from build123d import *

# Parameters (mm, degrees)
SKETCH1_R           = 61.976
SKETCH1_R_2         = 12.827
BOSS_EXTRUDE1_DEPTH = 45.974
SKETCH2_R           = 60.325
CUT_EXTRUDE1_DEPTH  = 20.32


with BuildPart() as part:
    # Sketch1 → Boss-Extrude1 (new body)
    with BuildSketch(Plane.XY):
        Circle(SKETCH1_R)
        Circle(SKETCH1_R_2, mode=Mode.SUBTRACT)
    extrude(amount=BOSS_EXTRUDE1_DEPTH)

    # Sketch2 → Cut-Extrude1 (cut)
    with BuildSketch(Plane.XY):
        Circle(SKETCH2_R)
    cut_extrude1 = extrude(amount=CUT_EXTRUDE1_DEPTH, mode=Mode.SUBTRACT)

    # Mirror1: Cut-Extrude1 across plane
    add(cut_extrude1.mirror(Plane.XY.offset(22.987)), mode=Mode.SUBTRACT)


solid = part.part
Verification items for the finished model (mm, model axes). A direction names the side the tool comes from. Coordinates: 2 decimals unless noted, no trailing zeros. Order: outer loops, then holes, each group sorted by start corner. A loop starts at its lowest first (then second) coordinate and runs counter-clockwise, first axis right, second up.
Item 1: Release check for a two-part mould opening along Z. For faces 4 (the face through (13.5, -59.4, 0)), 5 (the face through (12.235, 3.853, 22.95)), 6 (the face through (13.5, -59.4, 45.974)) record: +Z half, -Z half, draft (parallel to the pull), parting line (faces both ways), or undercut.
Filled in:
face 4: -Z half
face 5: draft
face 6: +Z half
Item 2: Access from +Z, -Z, +X, -X, +Y, -Y to the whole of each face (thin tool, end or side, straight path). Record for faces 1 (the face through (-60.267, 2.652, 35.956)), 2 (the face through (-60.267, 2.652, 10.018)), 3 (the face through (33.318, 52.258, 22.665)).
Filled in:
face 1: +Z
face 2: -Z
face 3: +Z, -Z
Item 3: Section check A-A, the plane x = 0. Enter the section's corners in (y, z) (3 decimals).
Filled in:
outline: (-61.976, 0) - (-60.325, 0) - (-60.325, 20.32) - (-12.827, 20.32) - (-12.827, 25.654) - (-60.325, 25.654) - (-60.325, 45.974) - (-61.976, 45.974) - close; (12.827, 20.32) - (60.325, 20.32) - (60.325, 0) - (61.976, 0) - (61.976, 45.974) - (60.325, 45.974) - (60.325, 25.654) - (12.827, 25.654) - close
Item 4: Section check C-C, the plane z = 23. Enter the section's corners in (x, y).
Filled in:
outline: circle Ø123.95 at (0, 0); hole circle Ø25.65 at (0, 0)
Item 5: Depth check by flat-ended pin: pin 1 (1.5 mm diameter, centred on x = 24, z = 39.5, fed in from -Y); pin 2 (4 mm diameter, centred on y = 11, z = 32.5, fed in from +X); pin 3 (4 mm diameter, centred on x = -33.5, y = 3.5, fed in from -Z). Enter the tip coordinate at first touch or a pass-through.
Filled in:
pin 1: stops at y = -57.45
pin 2: stops at x = 61.32
pin 3: stops at z = 20.32
Item 6: Section check D-D, the plane y = -21. Enter the section's corners in (x, z).
Filled in:
outline: (-58.31, 0) - (-56.55, 0) - (-56.55, 20.32) - (56.55, 20.32) - (56.55, 0) - (58.31, 0) - (58.31, 45.97) - (56.55, 45.97) - (56.55, 25.65) - (-56.55, 25.65) - (-56.55, 45.97) - (-58.31, 45.97) - close
Item 7: Material ranges on L1, parallel to Y at x = 0, z = 6.25 (3 decimals); L2, parallel to Z at x = -2, y = -24.5; L3, parallel to X at y = 21.5, z = 26, recorded low to high.
Filled in:
L1: y = -61.976 to -60.325, 60.325 to 61.976
L2: z = 20.32 to 25.65
L3: x = -58.13 to -56.36, 56.36 to 58.13
